from build123d import *

# Parameters (mm, degrees)
ESBO_O2_R             = 28.575
CORTE_EXTRUS_O1_DEPTH = 11.9126


with BuildPart() as part:
    # Esboço1 → Revolução1 (revolve)
    with BuildSketch(Plane.XY):
        Polygon((-11.9126, 0), (-11.9126, 14.5923), (-9.4996, 17.0053), (-2.413, 17.0053), (0, 14.5923), (0, 9.525), (85.09, 9.525), (86.03615, 8.57885), (86.03615, 0), align=None)
    revolve(axis=Axis((86.03615, 0, 0), (-1, 0, 0)))

    # Esboço2 → Corte-extrusão1 (cut)
    with BuildSketch(Plane(origin=(0, 0, 0), x_dir=(0, 0, -1), z_dir=(1, 0, 0))):
        Circle(ESBO_O2_R)
        Polygon((-14.2875, -8.248891971), (0, -16.497783942), (14.2875, -8.248891971), (14.2875, 8.248891971), (0, 16.497783942), (-14.2875, 8.248891971), align=None, mode=Mode.SUBTRACT)
    extrude(amount=-CORTE_EXTRUS_O1_DEPTH, mode=Mode.SUBTRACT)


solid = part.part
Work out the finished part from the listing and answer in its coordinate system (mm). A direction names the side the tool comes from. Round coordinates to 2 decimals unless told otherwise and drop trailing zeros. Loops run counter-clockwise (first coordinate to the right, second up) from the corner with the lowest first, then second, coordinate; pieces in that order, holes last. Notation, with made-up numbers: (29.25, -20) -> (73.25, -20) arc R11 cw to (73.25, -6) -> close; hole circle Ø11 at (51.25, -28.75). An arc over 180 degrees is marked (long way). Use one line per item in the form item = value.
(1) Flat-ended cylindrical pins translate along their axes: P1, Ø2, axis at x = 57, y = 0, coming from the -Z side (3 decimals); P2, Ø6, axis at x = 63, y = 9.5, coming from the +Z side; P3, Ø8, axis at x = 74.5, y = 5, coming from the +Z side. Find the tip coordinate at first contact, or state that the pin passes through.
Answer list:
P1 = -9.525
P2 = 6.96
P3 = 9.47
(2) A tool of negligible diameter and unlimited length cuts with its end or side. For faces 1 (the cylindrical face through (43.141, -7.559, 5.796)), 2 (the conical face through (-11.37, -15.135, -0.068)), from which of +Z, -Z, +X, -X, +Y, -Y can it reach the whole face along a straight path? Write none if from no direction.
Answer list:
face_1 = +X
face_2 = -X, -Y
(3) Find section A-A on y = 0. Give the vertices of the cut face in (x, z) (1 decimal), then the cut area to 3 significant figures.
Answer list:
outline = (-11.9, -14.3) -> (0, -14.3) -> (0, -9.5) -> (85.1, -9.5) -> (86, -8.6) -> (86, 8.6) -> (85.1, 9.5) -> (0, 9.5) -> (0, 14.3) -> (-11.9, 14.3) -> close
area = 1,980 mm2
(4) Straight lines are drawn through the part: line 1 (X direction, y = -6, z = 9.25); line 2 (Z direction, x = 18.5, y = 0.5); line 3 (Y direction, x = 79, z = 0.25). For each, find the intervals that lie inside material, in ascending order.
Answer list:
line_1 = -11.91 to 0
line_2 = -9.51 to 9.51
line_3 = -9.52 to 9.52
(5) Find section B-B on x = 36. Give the vertices of the cut face in (y, z) (3 decimals).
Answer list:
outline = circle Ø19.05 at (0, 0)
